Here's the drawing with two shaded views (mm, measured from the low corner). I have some questions. Give positions to 0.01 mm unless a question says otherwise; leave off trailing zeros. Write each loop counter-clockwise with the first axis right and the second up, starting at its lowest first coordinate (ties: lowest second). Pieces come first, ordered by that corner, then holes. Notation, with made-up numbers: (31, 9) - (90, 9) arc R33 ccw to (90, 43) - close; hole circle Ø11 at (49, -37). An arc over 180 degrees is marked (long way). Answer as a JSON object with one key per item and string values. Group by question number.
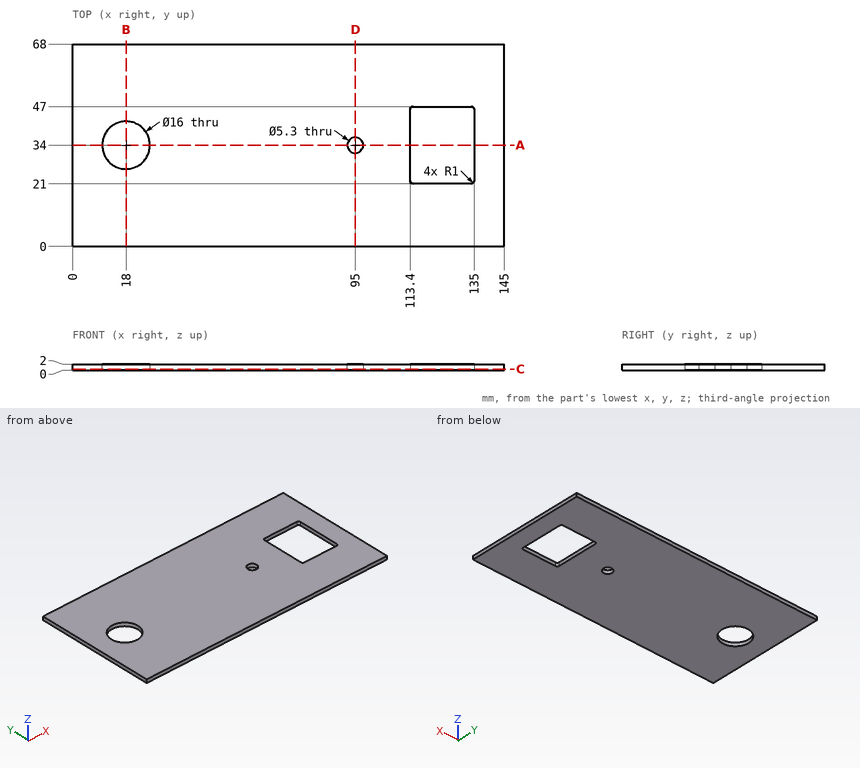
(1) I want a section at C-C, the plane z = 0.45. Please give me the cut outline in (x, y).
(2) I want a section at B-B, the plane x = 18. Please give me the cut outline in (y, z).
(3) I want a section at A-A, the plane y = 34. Please give me the cut outline in (x, z).
(4) I need wall thicknesses on L1, parallel to X at y = 23.5, z = 0.8; L2, parallel to Y at x = 18, z = 0.75; L3, parallel to Y at x = 95, z = 0.85. Which ranges of each line are inside material? Lowest first, please.
(5) I want a section at D-D, the plane x = 95. Please give me the cut outline in (y, z).
Entries:
{
 "1": {"outline": "(0, 0) - (145, 0) - (145, 68) - (0, 68) - close; hole circle Ø16 at (18, 34); hole circle Ø5.3 at (95, 34); hole (113.4, 22) arc R1 ccw to (114.4, 21) - (134, 21) arc R1 ccw to (135, 22) - (135, 46) arc R1 ccw to (134, 47) - (114.4, 47) arc R1 ccw to (113.4, 46) - close"},
 "2": {"outline": "(0, 0) - (26, 0) - (26, 2) - (0, 2) - close; (42, 0) - (68, 0) - (68, 2) - (42, 2) - close"},
 "3": {"outline": "(0, 0) - (10, 0) - (10, 2) - (0, 2) - close; (26, 0) - (92.35, 0) - (92.35, 2) - (26, 2) - close; (97.65, 0) - (113.4, 0) - (113.4, 2) - (97.65, 2) - close; (135, 0) - (145, 0) - (145, 2) - (135, 2) - close"},
 "4": {"L1": "0 to 113.4, 135 to 145", "L2": "0 to 26, 42 to 68", "L3": "0 to 31.35, 36.65 to 68"},
 "5": {"outline": "(0, 0) - (31.35, 0) - (31.35, 2) - (0, 2) - close; (36.65, 0) - (68, 0) - (68, 2) - (36.65, 2) - close"}
}
